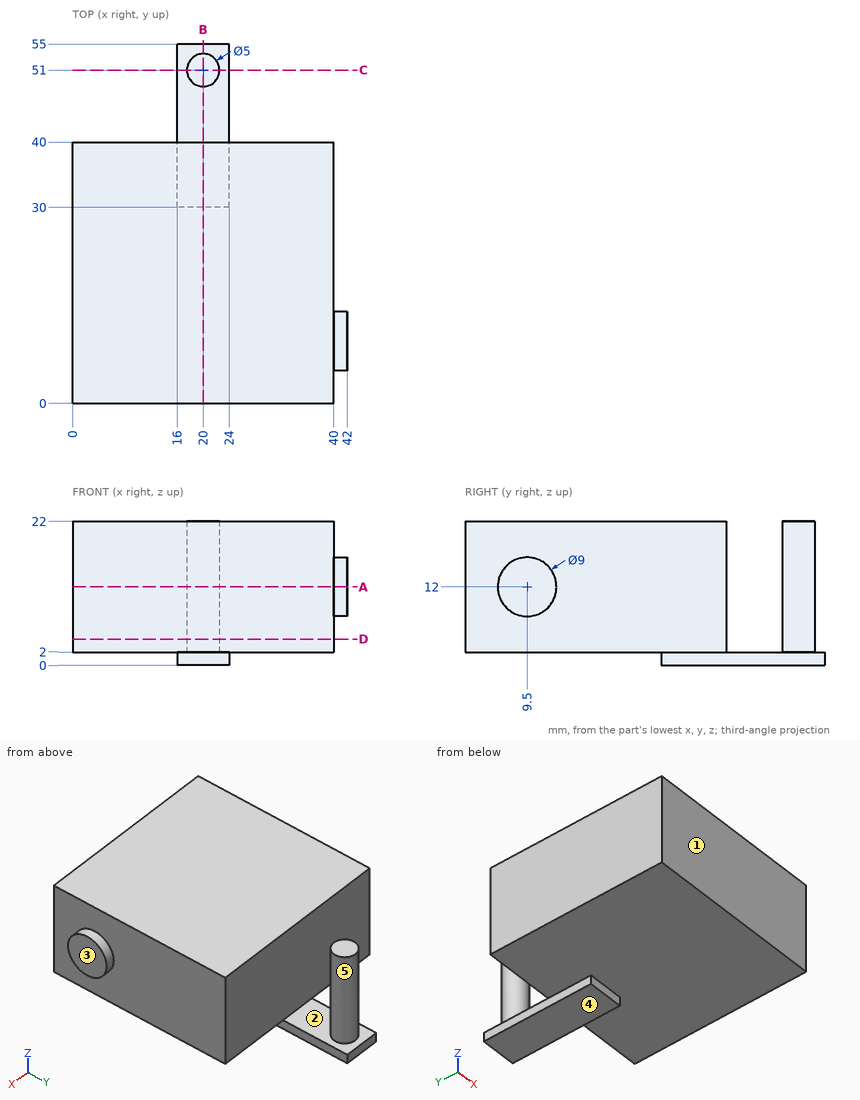
Answer from the drawing. Dimensions are ordinates in mm from the lowest x, y and z of the part. A direction names the side the tool comes from. Give positions to 0.01 mm unless a question says otherwise; leave off trailing zeros. Order: outer loops, then holes, each group sorted by start corner. A loop starts at its lowest first (then second) coordinate and runs counter-clockwise, first axis right, second up.
Item 1: The part is cut by section B-B, the plane x = 20. Give the vertices of the cut face in (y, z), and give its area (3 significant figures).
From the geometry:
outline: (0, 2) - (30, 2) - (30, 0) - (55, 0) - (55, 2) - (53.5, 2) - (53.5, 22) - (48.5, 22) - (48.5, 2) - (40, 2) - (40, 22) - (0, 22) - close
area: 950 mm2
Item 2: The part is cut by section D-D, the plane z = 4. Give the vertices of the cut face in (x, y), and give its area (3 significant figures).
From the geometry:
outline: (0, 0) - (40, 0) - (40, 40) - (0, 40) - close; circle Ø5 at (20, 51)
area: 1,620 mm2
Item 3: For a pull along Y with two mould halves and no side action, classify the marked faces 1, 2 and 3 as pulls with the +Y half, pulls with the -Y half, needs draft (parallel to the pull), parting line crosses it, or undercut.
From the geometry:
face 1: pulls with the -Y half
face 2: undercut
face 3: needs draft
Item 4: The part is cut by section A-A, the plane z = 12. Give the vertices of the cut face in (x, y).
From the geometry:
outline: (0, 0) - (40, 0) - (40, 5) - (42, 5) - (42, 14) - (40, 14) - (40, 40) - (0, 40) - close; circle Ø5 at (20, 51)
Item 5: Find the intervals of material crossed by probe 1 along X at (y, z) = (9, 5.5); probe 2 along Z at (x, y) = (34.5, 13), in increasing order.
From the geometry:
probe 1: x = 0 to 40
probe 2: z = 2 to 22
Item 6: The part is cut by section C-C, the plane y = 51. Give the vertices of the cut face in (x, z).
From the geometry:
outline: (16, 0) - (24, 0) - (24, 2) - (22.5, 2) - (22.5, 22) - (17.5, 22) - (17.5, 2) - (16, 2) - close
Item 7: Given pin 1 Ø4 at (y, z) = (44.5, 3.5) entering from -X; pin 2 Ø10 at (x, z) = (26, 13) entering from +Y; pin 3 Ø2 at (y, z) = (45, 1.5) entering from +X, each flat-ended and moving along its own axis, determine where each tip first touches the part or whether it passes through.
From the geometry:
pin 1: stops at x = 16
pin 2: stops at y = 53.29
pin 3: stops at x = 24
Item 8: Which of the six approach directions +Z, -Z, +X, -X, +Y, -Y give full straight-line access (tool end or side, diameter ignored) to the marked faces 4 and 5?
From the geometry:
face 4: -Z, +X, -X, +Y, -Y
face 5: +Z
